Read the model definition and answer for the solid it produces. Units are mm, in the model's axes. A direction names the side the tool comes from. Coordinates: 2 decimals unless noted, no trailing zeros. Loops run counter-clockwise (first coordinate to the right, second up) from the corner with the lowest first, then second, coordinate; pieces in that order, holes last. Notation, with made-up numbers: (82.25, 20) -> (92.25, 20) arc R14 ccw to (92.25, 39) -> close; hole circle Ø1 at (70, 88). An arc over 180 degrees is marked (long way). Answer as a JSON object with one key per item and string values. Group by question number.
1) Section D-D, the plane x = -19 is taken. Give the vertices of the cut face in (y, z), plus the area to 3 significant figures.
2) Determine the mould class of faces 1 (the face through (-20.341, 30, 5)), 2 (the face through (2.911, 80.568, 4.871)), 3 (the face through (19.409, 25, 3)), 4 (the face through (-25.091, 25, 3)) for opening direction X: released by +X, released by -X, zero draft, split by the parting line, or undercut.
3) Section A-A, the plane x = -14 is taken. Give the vertices of the cut face in (y, z).
4) Section B-B, the plane y = 63 is taken. Give the vertices of the cut face in (x, z).
5) Section C-C, the plane x = -4 is taken. Give the vertices of the cut face in (y, z).
6) Which of the six approach directions +Z, -Z, +X, -X, +Y, -Y give full straight-line access (tool end or side, diameter ignored) to faces 5 (the face through (-15.341, 30, 5)), 6 (the face through (-3, -33.969, 3)), 7 (the face through (9.659, 22, 5)), 8 (the face through (-3, 86.031, 3)), 9 (the face through (-8.593, -28.506, 4.871))?
7) Consider probe 1 along X at (y, z) = (38.5, 4.5); probe 2 along X at (y, z) = (79.5, 3.75); probe 3 along Y at (x, z) = (-10.5, 6.25). Determine where each line is inside the solid, lowest interval first. Write a range as [from, to].
from build123d import *

# Parameters (mm, degrees)
F0_W     = 44.5
F0_H     = 120
F1_DEPTH = 6.35
F3_DEPTH = 3


with BuildPart() as f1:
    # F0 (on Top) → F1 (new body)
    with BuildSketch(Plane.XY):
        with Locations((-2.840908, 26.030913)):
            Rectangle(F0_W, F0_H)
    extrude(amount=F1_DEPTH)

    # F2 (on face) → F3 (cut)
    with BuildSketch(Plane.XY.offset(6.35)):
        with BuildLine():
            Line((9.659092, 76.280913), (9.659092, -33.969087))
            Line((9.659092, -33.969087), (14.659092, -33.969087))
            Line((14.659092, -33.969087), (14.659092, 76.280913))
            Line((14.659092, 76.280913), (14.659092, 78.780913))
            ThreePointArc((14.659092, 78.780913), (13.926859, 80.548679), (12.159092, 81.280913))
            Line((12.159092, 81.280913), (4.659092, 81.280913))
            ThreePointArc((4.659092, 81.280913), (2.891325, 80.548679), (2.159092, 78.780913))
            Line((2.159092, 78.780913), (2.159092, -24.219087))
            Line((2.159092, -24.219087), (-0.340908, -24.219087))
            Line((-0.340908, -24.219087), (-0.340908, 78.780913))
            ThreePointArc((-0.340908, 78.780913), (-1.073141, 80.548679), (-2.840908, 81.280913))
            Line((-2.840908, 81.280913), (-10.340908, 81.280913))
            ThreePointArc((-10.340908, 81.280913), (-12.108675, 80.548679), (-12.840908, 78.780913))
            Line((-12.840908, 78.780913), (-12.840908, -24.219087))
            Line((-12.840908, -24.219087), (-15.340908, -24.219087))
            Line((-15.340908, -24.219087), (-15.340908, 86.030913))
            Line((-15.340908, 86.030913), (-20.340908, 86.030913))
            Line((-20.340908, 86.030913), (-20.340908, -26.719087))
            ThreePointArc((-20.340908, -26.719087), (-19.608675, -28.486854), (-17.840908, -29.219087))
            Line((-17.840908, -29.219087), (-10.340908, -29.219087))
            ThreePointArc((-10.340908, -29.219087), (-8.573141, -28.486854), (-7.840908, -26.719087))
            Line((-7.840908, -26.719087), (-7.840908, 76.280913))
            Line((-7.840908, 76.280913), (-5.340908, 76.280913))
            Line((-5.340908, 76.280913), (-5.340908, -26.719087))
            ThreePointArc((-5.340908, -26.719087), (-4.608675, -28.486854), (-2.840908, -29.219087))
            Line((-2.840908, -29.219087), (4.659092, -29.219087))
            ThreePointArc((4.659092, -29.219087), (6.426859, -28.486854), (7.159092, -26.719087))
            Line((7.159092, -26.719087), (7.159092, 76.280913))
            Line((7.159092, 76.280913), (9.659092, 76.280913))
        make_face()
    extrude(amount=-F3_DEPTH, mode=Mode.SUBTRACT)


solid = f1.part
Determined:
{
 "1": {"outline": "(-33.97, 0) -> (86.03, 0) -> (86.03, 3.35) -> (-28.93, 3.35) -> (-28.93, 6.35) -> (-33.97, 6.35) -> close", "area": "417 mm²"},
 "2": {"face 1": "undercut", "face 2": "undercut", "face 3": "released by +X", "face 4": "released by -X"},
 "3": {"outline": "(-33.97, 0) -> (86.03, 0) -> (86.03, 6.35) -> (-24.22, 6.35) -> (-24.22, 3.35) -> (-29.22, 3.35) -> (-29.22, 6.35) -> (-33.97, 6.35) -> close"},
 "4": {"outline": "(-25.09, 0) -> (19.41, 0) -> (19.41, 6.35) -> (14.66, 6.35) -> (14.66, 3.35) -> (9.66, 3.35) -> (9.66, 6.35) -> (7.16, 6.35) -> (7.16, 3.35) -> (2.16, 3.35) -> (2.16, 6.35) -> (-0.34, 6.35) -> (-0.34, 3.35) -> (-5.34, 3.35) -> (-5.34, 6.35) -> (-7.84, 6.35) -> (-7.84, 3.35) -> (-12.84, 3.35) -> (-12.84, 6.35) -> (-15.34, 6.35) -> (-15.34, 3.35) -> (-20.34, 3.35) -> (-20.34, 6.35) -> (-25.09, 6.35) -> close"},
 "5": {"outline": "(-33.97, 0) -> (86.03, 0) -> (86.03, 6.35) -> (81.28, 6.35) -> (81.28, 3.35) -> (-28.93, 3.35) -> (-28.93, 6.35) -> (-33.97, 6.35) -> close"},
 "6": {"face 5": "+Z, +Y", "face 6": "+Z, -Z, +X, -X, -Y", "face 7": "+Z, -Y", "face 8": "+Z, -Z, +X, -X, +Y", "face 9": "+Z"},
 "7": {"probe 1": "[-25.09, -20.34], [-15.34, -12.84], [-7.84, -5.34], [-0.34, 2.16], [7.16, 9.66], [14.66, 19.41]", "probe 2": "[-25.09, -20.34], [-15.34, -12.74], [-0.45, 2.26], [14.55, 19.41]", "probe 3": "[-33.97, -29.22], [81.28, 86.03]"}
}
